Source: three-view drawing plus pictorial views. Frame: mm from the lowest corner of the part. Coordinates: 2 decimals unless noted, no trailing zeros. Order: outer loops, then holes, each group sorted by start corner. A loop starts at its lowest first (then second) coordinate and runs counter-clockwise, first axis right, second up. Notation, with made-up numbers: (-22.75, 43) -> (18.25, 43) arc R21 ccw to (18.25, 49) -> close; hole circle Ø6 at (19, 69). An arc over 180 degrees is marked (long way). Use one line per item in the form item = value. Start each with the question number.
1) Section query C-C on z = 0.75. Count the separate pieces of the cut face and the enclosed holes in it, then the cut area to 3 significant figures.
2) Section query B-B on y = 30. Output: boundary loops of the cut face in (x, z).
3) Section query D-D on x = 27. Output: boundary loops of the cut face in (y, z), then the cut area to 3 significant figures.
4) Section query A-A on x = 34. Output: boundary loops of the cut face in (y, z).
5) Pin query (flat end, axial travel): pin 1 (6 mm diameter, centred on x = 21, y = 83.5, fed in from -Z). Return the tip coordinate at first contact, or that it passes through.
6) Ray query, line 1 along X through (y, z) = (110, 0.4); line 2 along X through (y, z) = (100, 1.3); line 3 along Y through (x, z) = (27, 1.5). Return the intervals inside material, ascending.
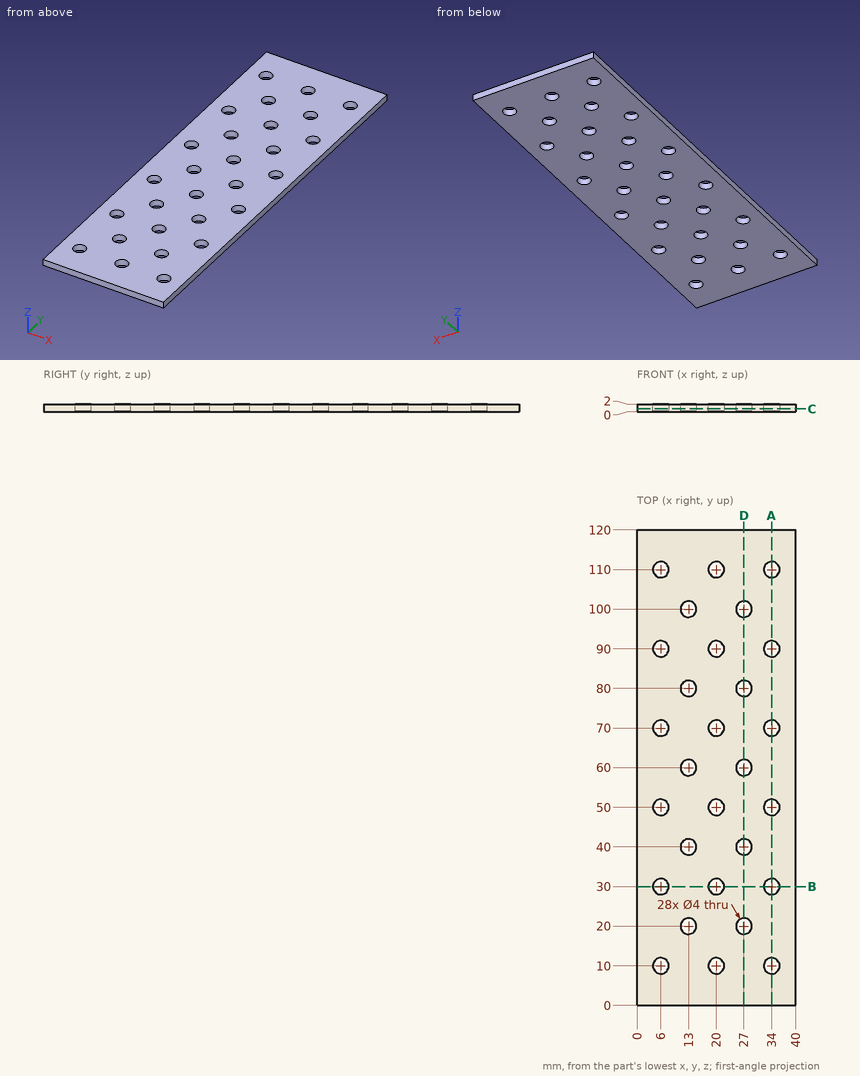
Answers below:
q1.separate_pieces = 1
q1.enclosed_holes = 28
q1.area = 4,450 mm^2
q2.outline = (0, 0) -> (4, 0) -> (4, 2) -> (0, 2) -> close; (8, 0) -> (18, 0) -> (18, 2) -> (8, 2) -> close; (22, 0) -> (32, 0) -> (32, 2) -> (22, 2) -> close; (36, 0) -> (40, 0) -> (40, 2) -> (36, 2) -> close
q3.outline = (0, 0) -> (18, 0) -> (18, 2) -> (0, 2) -> close; (22, 0) -> (38, 0) -> (38, 2) -> (22, 2) -> close; (42, 0) -> (58, 0) -> (58, 2) -> (42, 2) -> close; (62, 0) -> (78, 0) -> (78, 2) -> (62, 2) -> close; (82, 0) -> (98, 0) -> (98, 2) -> (82, 2) -> close; (102, 0) -> (120, 0) -> (120, 2) -> (102, 2) -> close
q3.area = 200 mm^2
q4.outline = (0, 0) -> (8, 0) -> (8, 2) -> (0, 2) -> close; (12, 0) -> (28, 0) -> (28, 2) -> (12, 2) -> close; (32, 0) -> (48, 0) -> (48, 2) -> (32, 2) -> close; (52, 0) -> (68, 0) -> (68, 2) -> (52, 2) -> close; (72, 0) -> (88, 0) -> (88, 2) -> (72, 2) -> close; (92, 0) -> (108, 0) -> (108, 2) -> (92, 2) -> close; (112, 0) -> (120, 0) -> (120, 2) -> (112, 2) -> close
q5.pin_1 = 0
q6.line_1 = 0 to 4, 8 to 18, 22 to 32, 36 to 40
q6.line_2 = 0 to 11, 15 to 25, 29 to 40
q6.line_3 = 0 to 18, 22 to 38, 42 to 58, 62 to 78, 82 to 98, 102 to 120
